```python
from build123d import *

# Parameters (mm, degrees)
F1_DEPTH = 12.7


with BuildPart() as f1:
    # F0 (on Front) → F1 (new body)
    with BuildSketch(Plane.XZ):
        Polygon((-49.171232, -6.599114), (-49.171232, 82.300886), (-41.551232, 82.300886), (-40.281232, 82.300886), (-32.661232, 82.300886), (-31.391232, 82.300886), (-23.771232, 82.300886), (-22.501232, 82.300886), (-14.881232, 82.300886), (-13.611232, 82.300886), (-5.991232, 82.300886), (-4.721232, 82.300886), (2.898768, 82.300886), (4.168768, 82.300886), (11.788768, 82.300886), (13.058768, 82.300886), (20.678768, 82.300886), (21.948768, 82.300886), (29.568768, 82.300886), (30.838768, 82.300886), (38.458768, 82.300886), (39.728768, 82.300886), (47.348768, 82.300886), (48.618768, 82.300886), (56.238768, 82.300886), (57.508768, 82.300886), (65.128768, 82.300886), (66.398768, 82.300886), (74.018768, 82.300886), (75.288768, 82.300886), (82.908768, 82.300886), (84.178768, 82.300886), (91.798768, 82.300886), (93.068768, 82.300886), (100.688768, 82.300886), (103.228768, 82.300886), (103.228768, 95.000886), (-61.871232, 95.000886), (-61.871232, -19.299114), (81.130768, -19.299114), (103.228768, -19.299114), (103.228768, -6.599114), (100.688768, -6.599114), (93.068768, -6.599114), (91.798768, -6.599114), (84.178768, -6.599114), (82.908768, -6.599114), (75.288768, -6.599114), (74.018768, -6.599114), (66.398768, -6.599114), (65.128768, -6.599114), (57.508768, -6.599114), (56.238768, -6.599114), (48.618768, -6.599114), (47.348768, -6.599114), (39.728768, -6.599114), (38.458768, -6.599114), (30.838768, -6.599114), (29.568768, -6.599114), (21.948768, -6.599114), (20.678768, -6.599114), (13.058768, -6.599114), (11.788768, -6.599114), (4.168768, -6.599114), (2.898768, -6.599114), (-4.721232, -6.599114), (-5.991232, -6.599114), (-13.611232, -6.599114), (-14.881232, -6.599114), (-22.501232, -6.599114), (-23.771232, -6.599114), (-31.391232, -6.599114), (-32.661232, -6.599114), (-40.281232, -6.599114), (-41.551232, -6.599114), align=None)
        Polygon((-41.551232, 82.300886), (-49.171232, 82.300886), (-45.361232, 75.701773), align=None)
        Polygon((-45.361232, 0), (-49.171232, -6.599114), (-41.551232, -6.599114), align=None)
        Polygon((-32.661232, 82.300886), (-40.281232, 82.300886), (-36.471232, 75.701773), align=None)
        Polygon((-36.471232, 0), (-40.281232, -6.599114), (-32.661232, -6.599114), align=None)
        Polygon((-23.771232, 82.300886), (-31.391232, 82.300886), (-27.581232, 75.701773), align=None)
        Polygon((-27.581232, 0), (-31.391232, -6.599114), (-23.771232, -6.599114), align=None)
        Polygon((-14.881232, 82.300886), (-22.501232, 82.300886), (-18.691232, 75.701773), align=None)
        Polygon((-18.691232, 0), (-22.501232, -6.599114), (-14.881232, -6.599114), align=None)
        Polygon((-5.991232, 82.300886), (-13.611232, 82.300886), (-9.801232, 75.701773), align=None)
        Polygon((-9.801232, 0), (-13.611232, -6.599114), (-5.991232, -6.599114), align=None)
        Polygon((2.898768, 82.300886), (-4.721232, 82.300886), (-0.911232, 75.701773), align=None)
        Polygon((-0.911232, 0), (-4.721232, -6.599114), (2.898768, -6.599114), align=None)
        Polygon((11.788768, 82.300886), (4.168768, 82.300886), (7.978768, 75.701773), align=None)
        Polygon((7.978768, 0), (4.168768, -6.599114), (11.788768, -6.599114), align=None)
        Polygon((20.678768, 82.300886), (13.058768, 82.300886), (16.868768, 75.701773), align=None)
        Polygon((16.868768, 0), (13.058768, -6.599114), (20.678768, -6.599114), align=None)
        Polygon((29.568768, 82.300886), (21.948768, 82.300886), (25.758768, 75.701773), align=None)
        Polygon((25.758768, 0), (21.948768, -6.599114), (29.568768, -6.599114), align=None)
        Polygon((38.458768, 82.300886), (30.838768, 82.300886), (34.648768, 75.701773), align=None)
        Polygon((34.648768, 0), (30.838768, -6.599114), (38.458768, -6.599114), align=None)
        Polygon((47.348768, 82.300886), (39.728768, 82.300886), (43.538768, 75.701773), align=None)
        Polygon((43.538768, 0), (39.728768, -6.599114), (47.348768, -6.599114), align=None)
        Polygon((56.238768, 82.300886), (48.618768, 82.300886), (52.428768, 75.701773), align=None)
        Polygon((52.428768, 0), (48.618768, -6.599114), (56.238768, -6.599114), align=None)
        Polygon((65.128768, 82.300886), (57.508768, 82.300886), (61.318768, 75.701773), align=None)
        Polygon((61.318768, 0), (57.508768, -6.599114), (65.128768, -6.599114), align=None)
        Polygon((74.018768, 82.300886), (66.398768, 82.300886), (70.208768, 75.701773), align=None)
        Polygon((70.208768, 0), (66.398768, -6.599114), (74.018768, -6.599114), align=None)
        Polygon((82.908768, 82.300886), (75.288768, 82.300886), (79.098768, 75.701773), align=None)
        Polygon((79.098768, 0), (75.288768, -6.599114), (82.908768, -6.599114), align=None)
        Polygon((91.798768, 82.300886), (84.178768, 82.300886), (87.988768, 75.701773), align=None)
        Polygon((87.988768, 0), (84.178768, -6.599114), (91.798768, -6.599114), align=None)
        Polygon((100.688768, 82.300886), (93.068768, 82.300886), (96.878768, 75.701773), align=None)
        Polygon((96.878768, 0), (93.068768, -6.599114), (100.688768, -6.599114), align=None)
    extrude(amount=F1_DEPTH)


solid = f1.part
```
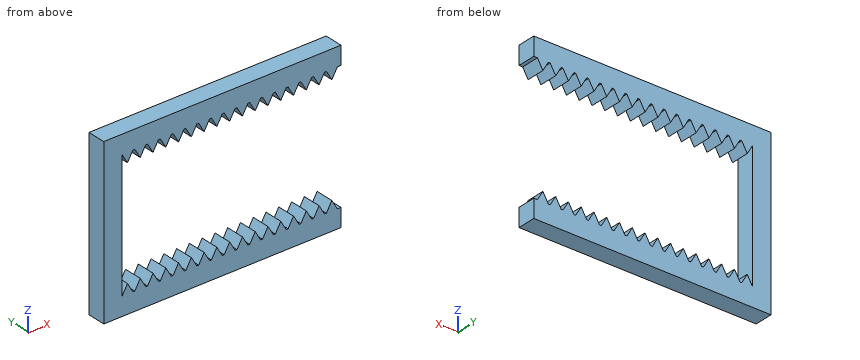
Here's how the part is built. I have some questions about the finished solid (model axes, mm). Coordinates: 2 decimals unless noted, no trailing zeros. Loops run counter-clockwise (first coordinate to the right, second up) from the corner with the lowest first, then second, coordinate; pieces in that order, holes last. Notation, with made-up numbers: (6, 58) -> (21, 58) arc R30 ccw to (21, 91) -> close; hole circle Ø2 at (-30.75, 39). An arc over 180 degrees is marked (long way). Return JSON: item names as keys, results as strings.
1) If we section it at B-B, the plane z = 71: Write out the boundary of the cut face in (x, y).
Results below:
{"outline": "(-61.87, -12.7) -> (-49.17, -12.7) -> (-49.17, 0) -> (-61.87, 0) -> close"}
2) Will these pins go through, and if not, where does the flat tip stop? pin 1 (2 mm diameter, centred on y = -7, z = 46, fed in from +X); pin 2 (1 mm diameter, centred on x = 8, z = 75, fed in from -Y).
Results below:
{"pin 1": "x = -49.17", "pin 2": "through"}
3) If we section it at C-C, the plane x = 45.5: Write out the boundary of the cut face in (y, z), then the cut area to 3 significant figures.
Results below:
{"outline": "(-12.7, -19.3) -> (0, -19.3) -> (0, -3.4) -> (-12.7, -3.4) -> close; (-12.7, 79.1) -> (0, 79.1) -> (0, 95) -> (-12.7, 95) -> close", "area": "404 mm²"}
4) I need wall thicknesses on line 1 (Z direction, x = -32.5, y = -3.5); line 2 (Z direction, x = -29.5, y = -11); line 3 (X direction, y = -0.5, z = 42). Which ranges of each line are inside material? Lowest first, please. Write a range as from..to.
Results below:
{"line 1": "-19.3..-6.6, 82.3..95", "line 2": "-19.3..-3.32, 79.03..95", "line 3": "-61.87..-49.17"}
5) If we section it at A-A, the plane x = -8: Write out the boundary of the cut face in (y, z), then the cut area to 3 significant figures.
Results below:
{"outline": "(-12.7, -19.3) -> (0, -19.3) -> (0, -3.12) -> (-12.7, -3.12) -> close; (-12.7, 78.82) -> (0, 78.82) -> (0, 95) -> (-12.7, 95) -> close", "area": "411 mm²"}
